from build123d import *

# Parameters (mm, degrees)
SKETCH_W        = 40
SKETCH_H        = 30
SKETCH_R        = 5.5
PAD_DEPTH       = 15
SKETCH001_R     = 8.15
POCKET_DEPTH    = 8
SKETCH002_R     = 2.6
POCKET001_DEPTH = 30.001


with BuildPart() as part:
    # Sketch → Pad (new body)
    with BuildSketch(Plane.XY):
        with Locations((0, -2)):
            Rectangle(SKETCH_W, SKETCH_H)
        Circle(SKETCH_R, mode=Mode.SUBTRACT)
    extrude(amount=PAD_DEPTH)

    # Sketch001 (on Face7 of Pad) → Pocket (cut)
    with BuildSketch(Plane.XY.offset(15)):
        Circle(SKETCH001_R)
    extrude(amount=-POCKET_DEPTH, mode=Mode.SUBTRACT)

    # Sketch002 (on Face1 of Pocket) → Pocket001 (cut, through all)
    with BuildSketch(Plane(origin=(0, 13, 0), x_dir=(-1, 0, 0), z_dir=(0, 1, 0))):
        with Locations((-12.5, 7.5)):
            Circle(SKETCH002_R)
        with Locations((12.5, 7.5)):
            Circle(SKETCH002_R)
    extrude(amount=-POCKET001_DEPTH, mode=Mode.SUBTRACT)


solid = part.part
Geometry: final body of the model. Coordinates: model frame, mm. A direction names the side the tool comes from. Round coordinates to 2 decimals unless told otherwise and drop trailing zeros. Loops run counter-clockwise (first coordinate to the right, second up) from the corner with the lowest first, then second, coordinate; pieces in that order, holes last. Notation, with made-up numbers: M 64.25,-10.75 L 123.25,-10.75 A27 ccw 123.25,20.25 Z; hole C -0.5,48.25 d6. An arc over 180 degrees is marked long. One line per question, with ' | ' between items.
(1) Pull-direction query (Z, two-part tool) for faces 3 (the cylindrical face through (10.1, -1.8, 6.5)), 4 (the cylindrical face through (-6.468, -4.959, 11.056)), 5 (the flat face through (-0.3, -8.5, 15)); classes: +Z half, -Z half, draft (parallel to the pull), parting line (faces both ways), or undercut.
Check result:
face 3: undercut | face 4: draft | face 5: +Z half
(2) Contact query for flat-ended pins moving along their axis: P1, Ø5, axis at x = 2, y = 2.5, coming from the +Z side; P2, Ø4.5, axis at x = 12.5, z = 7.5, coming from the +Y side. Output: stop coordinate, or through.
Check result:
P1: stops at z = 7 | P2: passes through
(3) Cut plane C-C on x = 0. Return the cut outline in (y, z), plus the area to 3 significant figures.
Check result:
outline: M -17,0 L -5.5,0 L -5.5,7 L -8.15,7 L -8.15,15 L -17,15 Z; M 5.5,0 L 13,0 L 13,15 L 8.15,15 L 8.15,7 L 5.5,7 Z | area: 243 mm2
(4) Cut plane A-A on z = 7.5. Return the cut outline in (x, y), plus the area to 3 significant figures.
Check result:
outline: M -20,-17 L -15.1,-17 L -15.1,13 L -20,13 Z; M -9.9,-17 L 9.9,-17 L 9.9,13 L -9.9,13 Z; M 15.1,-17 L 20,-17 L 20,13 L 15.1,13 Z; hole C 0,0 d16.3 | area: 679 mm2
(5) Access query for faces 1 (the flat face through (0, -17, 7)), 2 (the flat face through (5.32, 1.93, 7)). Directions: +Z, -Z, +X, -X, +Y, -Y. A direction counts if a zero-diameter tool reaches every point of the face in a straight line with its end or side. Return the directions, or none.
Check result:
face 1: +Z, -Z, +X, -X, -Y | face 2: +Z
(6) Material intervals for line 1 along Z through (x, y) = (-12.5, 1.5); line 2 along X through (y, z) = (-8, 6.75); line 3 along Y through (x, z) = (0, 3.5), sorted ascending. Write a range as from..to.
Check result:
line 1: z = 0..4.9, 10.1..15 | line 2: x = -20..-14.99, -10.01..10.01, 14.99..20 | line 3: y = -17..-5.5, 5.5..13
(7) Cut plane B-B on y = 0. Return the cut outline in (x, z).
Check result:
outline: M -20,0 L -5.5,0 L -5.5,7 L -8.15,7 L -8.15,15 L -20,15 Z; M 5.5,0 L 20,0 L 20,15 L 8.15,15 L 8.15,7 L 5.5,7 Z; hole C -12.5,7.5 d5.2; hole C 12.5,7.5 d5.2
(8) Cut plane D-D on z = 14.25. Return the cut outline in (x, y), plus the area to 3 significant figures.
Check result:
outline: M -20,-17 L 20,-17 L 20,13 L -20,13 Z; hole C 0,0 d16.3 | area: 991 mm2
